Input: part model. Units: mm. Frame: model coordinates. A direction names the side the tool comes from. Give positions to 0.01 mm unless a question says otherwise; leave off trailing zeros. Write each loop counter-clockwise with the first axis right and the second up, starting at its lowest first coordinate (ties: lowest second). Pieces come first, ordered by that corner, then holes. Notation, with made-up numbers: (-22.5, 34) - (-2.5, 34) arc R22 cw to (-2.5, 46) - close; hole circle Ø11 at (2, 23). An arc over 180 degrees is marked (long way). Answer as CSV lines item,"result".
```python
from build123d import *

# Parameters (mm, degrees)
SKETCH4_R                       = 33
CUT_EXTRUDE1_DEPTH              = 2
M3X0_5_TAPPED_HOLE1_D           = 2.5
M3X0_5_TAPPED_HOLE1_DEPTH       = 7.5
M3X0_5_TAPPED_HOLE1_TIP         = 0.751075774
M3X0_5_TAPPED_HOLE2_D           = 2.5
M3X0_5_TAPPED_HOLE2_DEPTH       = 7.5
M3X0_5_TAPPED_HOLE2_CSINK_D     = 3.05
M3X0_5_TAPPED_HOLE2_CSINK_ANGLE = 90
M3X0_5_TAPPED_HOLE2_TIP         = 0.751075774


with BuildPart() as part:
    # Sketch3 → Revolve1 (revolve)
    with BuildSketch(Plane.XY):
        Polygon((0, -10.05), (0, 10.05), (18.5, 10.05), (34, 5.55), (34, -10.05), align=None)
    revolve(axis=Axis((0, -10.05, 0), (0, 1, 0)))

    # Sketch4 → Cut-Extrude1 (cut)
    with BuildSketch(Plane.XZ.offset(10.05)):
        Circle(SKETCH4_R)
    extrude(amount=-CUT_EXTRUDE1_DEPTH, mode=Mode.SUBTRACT)

    # M3x0.5 Tapped Hole1
    with Locations(Plane(origin=(0, 10.05, 0), x_dir=(1, 0, 0), z_dir=(0, 1, 0))):
        with Locations((-10.606601718, 10.606601718), (10.606601718, 10.606601718), (10.606601718, -10.606601718), (-10.606601718, -10.606601718)):
            Hole(M3X0_5_TAPPED_HOLE1_D / 2, depth=M3X0_5_TAPPED_HOLE1_DEPTH)
            with Locations((0, 0, -(M3X0_5_TAPPED_HOLE1_DEPTH + M3X0_5_TAPPED_HOLE1_TIP / 2))):  # 118° drill point
                Cone(0, M3X0_5_TAPPED_HOLE1_D / 2, M3X0_5_TAPPED_HOLE1_TIP, mode=Mode.SUBTRACT)

    # M3x0.5 Tapped Hole2
    with Locations(Plane(origin=(0, 10.05, 0), x_dir=(1, 0, 0), z_dir=(0, 1, 0))):
        with Locations((0, 12.5), (0, -12.5), (-12.5, 0), (12.5, 0)):
            CounterSinkHole(M3X0_5_TAPPED_HOLE2_D / 2, M3X0_5_TAPPED_HOLE2_CSINK_D / 2, depth=M3X0_5_TAPPED_HOLE2_DEPTH, counter_sink_angle=M3X0_5_TAPPED_HOLE2_CSINK_ANGLE)
            with Locations((0, 0, -(M3X0_5_TAPPED_HOLE2_DEPTH + M3X0_5_TAPPED_HOLE2_TIP / 2))):  # 118° drill point
                Cone(0, M3X0_5_TAPPED_HOLE2_D / 2, M3X0_5_TAPPED_HOLE2_TIP, mode=Mode.SUBTRACT)


solid = part.part
```
Item 1: Reachability of faces 3 (the face through (-11.25, 6.11, -0.05)), 4 (the face through (0, -8.05, 0)) from +Z, -Z, +X, -X, +Y, -Y: full face, straight path, thin tool, end or side. Return the list, or none.
The answers:
face 3,"+Y"
face 4,"-Y"
Item 2: Contact query for flat-ended pins moving along their axis: pin 1 (2 mm diameter, centred on x = -10.61, z = 10.61, fed in from +Y); pin 2 (4 mm diameter, centred on x = 0, z = -12.5, fed in from -Y); pin 3 (1 mm diameter, centred on x = 26, y = 5.5, fed in from +Z); pin 4 (3 mm diameter, centred on x = -10.61, z = -10.61, fed in from +Y). Output: stop coordinate, or through.
The answers:
pin 1,"y = 2.4"
pin 2,"y = -8.05"
pin 3,"z = 22.49"
pin 4,"y = 10.05"
Item 3: Ray query, line 1 (Z direction, x = 0, y = -8.8); line 2 (Y direction, x = 12.5, z = 8); line 3 (X direction, y = -8.25, z = -4). Return the intervals inside material, ascending. Write a range as from..to.
The answers:
line 1,"-34..-33, 33..34"
line 2,"-8.05..10.05"
line 3,"-33.76..-32.76, 32.76..33.76"
Item 4: Mould query, pull axis Z, two halves, no side actions, for faces 1 (the face through (18.28, -2.36, -28.67)), 2 (the face through (0.16, 6.11, -13.74)). Classes: +Z half, -Z half, draft (parallel to the pull), parting line (faces both ways), or undercut.
The answers:
face 1,"parting line"
face 2,"undercut"
Item 5: Cut plane A-A on y = -4.5. Return the cut outline in (x, z).
The answers:
outline,"circle Ø68 at (0, 0)"
